Input: dimensioned drawing with shaded views. Units: mm. Origin: part minimum x, y, z. Round coordinates to 2 decimals unless told otherwise and drop trailing zeros. Order: outer loops, then holes, each group sorted by start corner. A loop starts at its lowest first (then second) coordinate and runs counter-clockwise, first axis right, second up.
Item 1: Cut plane B-B on z = 1.75. Output: boundary loops of the cut face in (x, y), then the cut area to 3 significant figures.
Item 2: First-contact query: pin 1 (2.5 mm diameter, centred on x = 5, y = 21.5, fed in from +Z). Flat tip, straight axial feed; report the tip coordinate or a pass-through.
Item 3: Cut plane A-A on x = 45. Output: boundary loops of the cut face in (y, z), then the cut area to 3 significant figures.
Item 4: Cut plane C-C on y = 21.5. Output: boundary loops of the cut face in (x, z).
Item 5: Cut plane D-D on x = 23. Output: boundary loops of the cut face in (y, z), then the cut area to 3 significant figures.
Item 6: Line query: L1, parallel to Y at x = 5, z = 2; L2, parallel to Y at x = 21.5, z = 1.05; L3, parallel to X at y = 26, z = 1.2. Output: solid intervals per line, ascending.
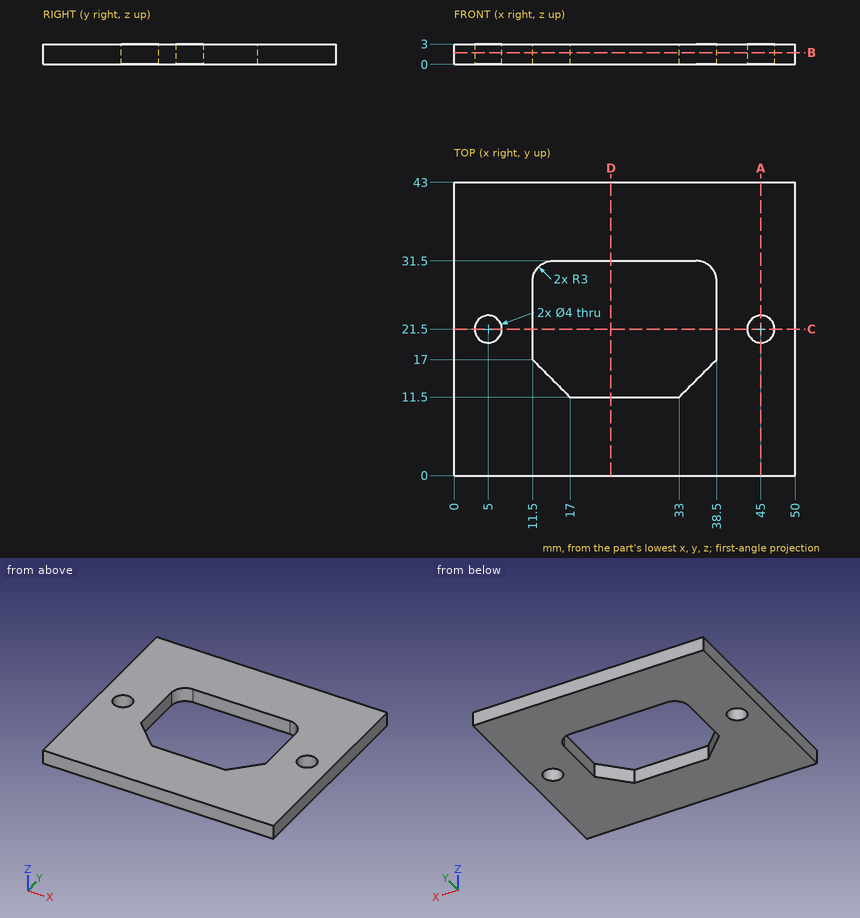
From the geometry:
1. outline: (0, 0) - (50, 0) - (50, 43) - (0, 43) - close; hole circle Ø4 at (5, 21.5); hole (11.5, 17) - (17, 11.5) - (33, 11.5) - (38.5, 17) - (38.5, 28.5) arc R3 ccw to (35.5, 31.5) - (14.5, 31.5) arc R3 ccw to (11.5, 28.5) - close; hole circle Ø4 at (45, 21.5)
1. area: 1,620 mm2
2. pin 1: passes through
3. outline: (0, 0) - (19.5, 0) - (19.5, 3) - (0, 3) - close; (23.5, 0) - (43, 0) - (43, 3) - (23.5, 3) - close
3. area: 117 mm2
4. outline: (0, 0) - (3, 0) - (3, 3) - (0, 3) - close; (7, 0) - (11.5, 0) - (11.5, 3) - (7, 3) - close; (38.5, 0) - (43, 0) - (43, 3) - (38.5, 3) - close; (47, 0) - (50, 0) - (50, 3) - (47, 3) - close
5. outline: (0, 0) - (11.5, 0) - (11.5, 3) - (0, 3) - close; (31.5, 0) - (43, 0) - (43, 3) - (31.5, 3) - close
5. area: 69.0 mm2
6. L1: y = 0 to 19.5, 23.5 to 43
6. L2: y = 0 to 11.5, 31.5 to 43
6. L3: x = 0 to 11.5, 38.5 to 50
